Could you check a few things on this model? Use its own coordinates, in mm. Face numbers are marked on the shaded views. A direction names the side the tool comes from. Coordinates: 2 decimals unless noted, no trailing zeros. Loops run counter-clockwise (first coordinate to the right, second up) from the corner with the lowest first, then second, coordinate; pieces in that order, holes last. Notation, with made-up numbers: (68, 32.5) -> (118, 32.5) arc R14 ccw to (118, 52.5) -> close; hole circle Ø7 at (25, 89.5). An arc over 180 degrees is marked (long way). One line per question, with ' | ' between items.
```python
from build123d import *

# Parameters (mm, degrees)
SKETCH1_R           = 2
BOSS_EXTRUDE1_DEPTH = 9.4
SKETCH2_W           = 6
SKETCH2_H           = 0.5
CUT_EXTRUDE1_DEPTH  = 8
SKETCH3_R           = 3.5
BOSS_EXTRUDE2_DEPTH = 2.6
SKETCH4_R           = 12.5
SKETCH4_R_2         = 12.4
EXTRUDE_THIN1_DEPTH = 67
SKETCH6_R           = 12.5
BOSS_EXTRUDE4_DEPTH = 0.1
BOSS_EXTRUDE5_START = -0.1
SKETCH7_R           = 12.5
BOSS_EXTRUDE5_DEPTH = 0.1


with BuildPart() as part:
    # Sketch1 → Boss-Extrude1 (new body)
    with BuildSketch(Plane.XY):
        Circle(SKETCH1_R)
    extrude(amount=-BOSS_EXTRUDE1_DEPTH)

    # Sketch2 → Cut-Extrude1 (cut)
    with BuildSketch(Plane.XY):
        with Locations((0.35899941, -1.75)):
            Rectangle(SKETCH2_W, SKETCH2_H)
    extrude(amount=-CUT_EXTRUDE1_DEPTH, mode=Mode.SUBTRACT)

    # Sketch3 → Boss-Extrude2 (add)
    with BuildSketch(Plane(origin=(0, 0, -9.4), x_dir=(-1, 0, 0), z_dir=(0, 0, -1))):
        Circle(SKETCH3_R)
    extrude(amount=BOSS_EXTRUDE2_DEPTH)



with BuildPart() as body_2:
    # Sketch4 → Extrude-Thin1 (new body)
    with BuildSketch(Plane(origin=(0, 0, -12), x_dir=(-1, 0, 0), z_dir=(0, 0, -1))):
        Circle(SKETCH4_R)
        Circle(SKETCH4_R_2, mode=Mode.SUBTRACT)
    extrude(amount=EXTRUDE_THIN1_DEPTH)


with BuildPart() as part_1:
    add(part.part)

    add(body_2.part)  # Boss-Extrude4 merges body 2
    # Sketch6 → Boss-Extrude4 (add)
    with BuildSketch(Plane(origin=(0, 0, -12), x_dir=(-1, 0, 0), z_dir=(0, 0, -1))):
        Circle(SKETCH6_R)
    extrude(amount=BOSS_EXTRUDE4_DEPTH)

    # Sketch7 → Boss-Extrude5 (add)
    with BuildSketch(Plane(origin=(0, 0, -79), x_dir=(-1, 0, 0), z_dir=(0, 0, -1)).offset(BOSS_EXTRUDE5_START)):
        Circle(SKETCH7_R)
    extrude(amount=BOSS_EXTRUDE5_DEPTH)


solid = part_1.part
```
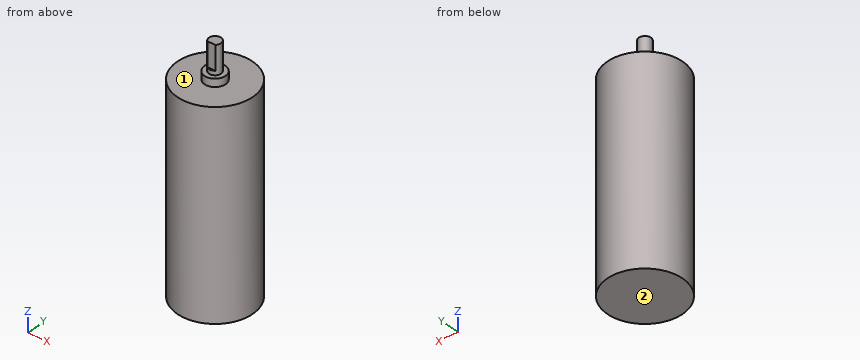
Q1. Imagine slicing it at A-A on y = 0. Write out the boundary of the cut face in (x, z), plus the area to 3 significant figures.
Values follow:
outline: (-12.5, -79) -> (12.5, -79) -> (12.5, -12) -> (3.5, -12) -> (3.5, -9.4) -> (2, -9.4) -> (2, 0) -> (-2, 0) -> (-2, -9.4) -> (-3.5, -9.4) -> (-3.5, -12) -> (-12.5, -12) -> close; hole (-12.4, -78.9) -> (12.4, -78.9) -> (12.4, -12.1) -> (-12.4, -12.1) -> close | area: 74.2 mm2
Q2. For pin 1 (8 mm diameter, centred on x = 8, z = -53, fed in from +Y); pin 2 (1.5 mm diameter, centred on y = -2.5, z = -21, fed in from -X); pin 3 (2 mm diameter, centred on x = 0, z = -4, fed in from -Y); pin 4 (12.5 mm diameter, centred on x = 3, y = -2.5, fed in from +Z), each with a flat end and sliding along its axis, tell me the tip position at first contact or that it passes through.
Values follow:
pin 1: stops at y = 11.84 | pin 2: stops at x = -12.38 | pin 3: stops at y = -1.5 | pin 4: stops at z = 0
Q3. Imagine slicing it at B-B on x = 0. Write out the boundary of the cut face in (y, z).
Values follow:
outline: (-12.5, -79) -> (12.5, -79) -> (12.5, -12) -> (3.5, -12) -> (3.5, -9.4) -> (2, -9.4) -> (2, 0) -> (-1.5, 0) -> (-1.5, -8) -> (-2, -8) -> (-2, -9.4) -> (-3.5, -9.4) -> (-3.5, -12) -> (-12.5, -12) -> close; hole (-12.4, -78.9) -> (12.4, -78.9) -> (12.4, -12.1) -> (-12.4, -12.1) -> close
Q4. Imagine slicing it at C-C on z = -53. Write out the boundary of the cut face in (x, y), plus the area to 3 significant figures.
Values follow:
outline: circle Ø25 at (0, 0); hole circle Ø24.8 at (0, 0) | area: 7.82 mm2
Q5. For the marked faces 1 and 2, which set-ups out of +Z, -Z, +X, -X, +Y, -Y let a thin tool reach every point of the face, with its end or its side?
Values follow:
face 1: +Z | face 2: -Z, +X, -X, +Y, -Y
Q6. Please list where these lines run through material, in increasing order: L1, parallel to X at y = -10, z = -75.5; L2, parallel to Y at x = -11, z = -51; L3, parallel to Y at x = 0.75, z = -8.5. Write a range as [from, to].
Values follow:
L1: x = [-7.5, -7.33], [7.33, 7.5] | L2: y = [-5.94, -5.72], [5.72, 5.94] | L3: y = [-1.85, 1.85]
